Verification items for the finished model (mm, model axes). Face numbers are marked on the shaded views. A direction names the side the tool comes from. Round coordinates to 2 decimals unless told otherwise and drop trailing zeros. Order: outer loops, then holes, each group sorted by start corner. A loop starts at its lowest first (then second) coordinate and runs counter-clockwise, first axis right, second up. Notation, with made-up numbers: M 39,89.25 L 82,89.25 A14 ccw 82,94.25 Z; hole C 15.25,85.5 d10. An arc over 180 degrees is marked long. Write item = value, one per line. Start each with the question number.
from build123d import *

# Parameters (mm, degrees)
SKETCH8_W           = 70
SKETCH8_H           = 36
BOSS_EXTRUDE3_DEPTH = 3
SKETCH9_W           = 6
SKETCH9_H           = 32
BOSS_EXTRUDE4_DEPTH = 20.47521
CUT_EXTRUDE1_DEPTH  = 100
BOSS_EXTRUDE5_DEPTH = 3
BOSS_EXTRUDE6_DEPTH = 70
SKETCH15_R          = 1.3
CUT_EXTRUDE2_DEPTH  = 3
CUT_EXTRUDE3_DEPTH  = 100
SKETCH17_W          = 62
SKETCH17_H          = 10
CUT_EXTRUDE4_DEPTH  = 1
FILLET1_R           = 1
CUT_EXTRUDE5_DEPTH  = 10


with BuildPart() as part:
    # Sketch8 → Boss-Extrude3 (new body)
    with BuildSketch(Plane(origin=(0, 0, 0), x_dir=(1, 0, 0), z_dir=(0, 1, 0))):
        with Locations((35, 18)):
            Rectangle(SKETCH8_W, SKETCH8_H)
    extrude(amount=BOSS_EXTRUDE3_DEPTH)

    # Sketch9 → Boss-Extrude4 (add)
    with BuildSketch(Plane(origin=(0, 3, 0), x_dir=(1, 0, 0), z_dir=(0, 1, 0))):
        with Locations((61, 20)):
            Rectangle(SKETCH9_W, SKETCH9_H)
        with Locations((9, 20)):
            Rectangle(SKETCH9_W, SKETCH9_H)
        with Locations((35, 20)):
            Rectangle(SKETCH9_W, SKETCH9_H)
    extrude(amount=BOSS_EXTRUDE4_DEPTH)

    # Sketch10 → Cut-Extrude1 (cut)
    with BuildSketch(Plane.ZY.offset(-6)):
        Polygon((-36, 5), (-4, 23.47521), (-36, 23.47521), align=None)
    extrude(amount=-CUT_EXTRUDE1_DEPTH, mode=Mode.SUBTRACT)

    # Sketch11 → Boss-Extrude5 (add)
    with BuildSketch(Plane(origin=(0, 19.338457712, -11.165064603), x_dir=(1, 0, 0), z_dir=(0, 0.8660253875430481, -0.5000000281309126))):
        Polygon((6, 38.676913811), (-5, 38.676913811), (-5, -11.323086189), (75, -11.323086189), (75, 38.676913811), (64, 38.676913811), align=None)
    extrude(amount=BOSS_EXTRUDE5_DEPTH)

    # Sketch14 → Boss-Extrude6 (add)
    with BuildSketch(Plane.ZY):
        Polygon((-36, 0), (-44.660253875, -2.81e-07), (-36, 5), align=None)
    extrude(amount=-BOSS_EXTRUDE6_DEPTH)

    # Sketch15 → Cut-Extrude2 (cut)
    with BuildSketch(Plane(origin=(0, 21.936533875, -12.665064688), x_dir=(1, 0, 0), z_dir=(0, 0.8660253875430481, -0.5000000281309125))):
        with Locations(Location((-3, 36.676913811, 0), (0, 0, 270))):
            Circle(SKETCH15_R)
        with Locations(Location((73, 36.676913811, 0), (0, 0, 90))):
            Circle(SKETCH15_R)
        with Locations(Location((73, -9.323086189, 0), (0, 0, 270))):
            Circle(SKETCH15_R)
        with Locations(Location((-3, -9.323086189, 0), (0, 0, 90))):
            Circle(SKETCH15_R)
    extrude(amount=-CUT_EXTRUDE2_DEPTH, mode=Mode.SUBTRACT)

    # Sketch16 → Cut-Extrude3 (cut)
    with BuildSketch(Plane.ZY.offset(-6)):
        Polygon((-7, 6), (-7, 18.279057382), (-28.26794966, 6), align=None)
    extrude(amount=-CUT_EXTRUDE3_DEPTH, mode=Mode.SUBTRACT)

    # Sketch17 → Cut-Extrude4 (cut)
    with BuildSketch(Plane.XZ):
        with Locations((35, -7)):
            Rectangle(SKETCH17_W, SKETCH17_H)
        with Locations((35, -37.660253875)):
            Rectangle(SKETCH17_W, SKETCH17_H)
    extrude(amount=-CUT_EXTRUDE4_DEPTH, mode=Mode.SUBTRACT)

    # Fillet1
    fillet1_edges = [part.edges().sort_by_distance(p)[0] for p in [
        (70, 1.5, 0),
        (0, 1.5, 0),
        (-5, 1.2990378, -45.410253918),
        (-5, 26.299039207, -2.10898454),
        (75, 26.299039207, -2.10898454),
        (75, 1.2990378, -45.410253918),
    ]]
    fillet(fillet1_edges, radius=FILLET1_R)

    # Sketch18 → Cut-Extrude5 (cut)
    with BuildSketch(Plane(origin=(0, 19.338457712, -11.165064603), x_dir=(1, 0, 0), z_dir=(0, -0.8660253875430481, 0.5000000281309125))):
        with BuildLine():
            Line((49.57742676, 6.27350411), (49.57742676, 9.27350411))
            Line((49.57742676, 9.27350411), (52.28871338, 11.323086189))
            Line((52.28871338, 11.323086189), (53.28871338, 11.323086189))
            Line((53.28871338, 11.323086189), (56, 9.27350411))
            Line((56, 9.27350411), (56, 6.27350411))
            Line((56, 6.27350411), (56, 3.12980455))
            ThreePointArc((56, 3.12980455), (55.707106781, 2.422697769), (55, 2.12980455))
            Line((55, 2.12980455), (50.57742676, 2.12980455))
            ThreePointArc((50.57742676, 2.12980455), (49.870319979, 2.422697769), (49.57742676, 3.12980455))
            Line((49.57742676, 3.12980455), (49.57742676, 6.27350411))
        make_face()
    extrude(amount=-CUT_EXTRUDE5_DEPTH, mode=Mode.SUBTRACT)


solid = part.part
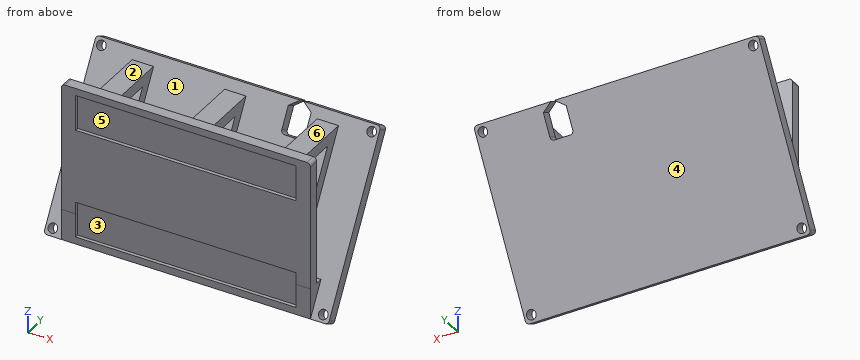
1) Scan lines: probe 1 along X at (y, z) = (19.75, -10); probe 2 along X at (y, z) = (24.25, -7.5); probe 3 along Y at (x, z) = (49.5, -32.5). Record each from-to range of solid material in increasing order.
2) Cross-section at A-A, the plane x = 68. Enter the section's corners in (y, z).
3) Access from +Z, -Z, +X, -X, +Y, -Y to the whole of each face (thin tool, end or side, straight path). Record for the marked faces 1, 2 and 3.
4) Gauge pin test, flat ends, axial feed: P1, Ø6.5, axis at x = 34, z = -21.5, coming from the +Y side; P2, Ø10, axis at x = 49.5, y = 20, coming from the -Z side; P3, Ø1.5, axis at x = 35, z = -16, coming from the +Y side. Record the tip position at first contact, or that the pin passes through.
5) Cross-section at C-C, the plane y = 9.5. Enter the section's corners in (x, z), then the cut area to 3 significant figures.
6) Cross-section at B-B, the plane z = -31.5. Enter the section's corners in (x, y).
7) Cross-section at D-D, the plane x = 36. Enter the section's corners in (y, z), then the cut area to 3 significant figures.
8) Release check for a two-part mould opening along Y. For the marked faces 4, 5 and 6 record: pulls with the +Y half, pulls with the -Y half, needs draft (parallel to the pull), parting line crosses it, or undercut.
Geometry results:
q1.probe_1 = 6 to 12, 32 to 38, 58 to 64
q1.probe_2 = -5 to 49.58, 56 to 75
q1.probe_3 = 0 to 3, 7.02 to 10.48
q2.outline = M 0,-44.66 L 2.6,-46.16 L 27.6,-2.86 L 25,-1.36 L 5,-36 L 3,-36 L 3,0 L 0,0 Z
q3.face_1 = +Z
q3.face_2 = +Z, +X, -X
q3.face_3 = -Y
q4.P1 = 18.71
q4.P2 = -24.68
q4.P3 = 20.44
q5.outline = M -5,-34.21 L 75,-34.21 L 75,-28.21 L 64,-28.21 L 64,-22.21 L 58,-22.21 L 58,-28.21 L 38,-28.21 L 38,-22.21 L 32,-22.21 L 32,-28.21 L 12,-28.21 L 12,-22.21 L 6,-22.21 L 6,-28.21 L -5,-28.21 Z; M 6,-7 L 12,-7 L 12,-4 L 6,-4 Z; M 32,-7 L 38,-7 L 38,-4 L 32,-4 Z; M 58,-7 L 64,-7 L 64,-4 L 58,-4 Z
q5.area = 642 mm^2
q6.outline = M -5,7.6 L 6,7.6 L 6,3 L 0,3 L 0,0 L 70,0 L 70,3 L 64,3 L 64,7.6 L 75,7.6 L 75,11.06 L -5,11.06 Z; hole M 12,3 L 32,3 L 32,7.6 L 12,7.6 Z; hole M 38,3 L 58,3 L 58,7.6 L 38,7.6 Z
q7.outline = M 0,-44.66 L 2.6,-46.16 L 27.6,-2.86 L 25,-1.36 L 23.48,-4 L 3,-4 L 3,0 L 0,0 L 0,-2 L 1,-2 L 1,-12 L 0,-12 L 0,-32.66 L 1,-32.66 L 1,-42.66 L 0,-42.66 Z; hole M 6,-28.27 L 18.28,-7 L 6,-7 Z
q7.area = 489 mm^2
q8.face_4 = pulls with the +Y half
q8.face_5 = pulls with the -Y half
q8.face_6 = undercut
